Read the model definition and answer for the solid it produces. Units are mm, in the model's axes. A direction names the side the tool comes from. Coordinates: 2 decimals unless noted, no trailing zeros. Order: outer loops, then holes, each group sorted by start corner. A loop starts at its lowest first (then second) coordinate and runs counter-clockwise, first axis right, second up. Notation, with made-up numbers: (47.25, -7) -> (78.25, -7) arc R14 ccw to (78.25, 6) -> close; hole circle Ø8 at (39, -36.5). An arc over 180 degrees is marked (long way). Use CSV: the item, a comma, the result in double quotes.
```python
from build123d import *

# Parameters (mm, degrees)
F0_R     = 20
F0_R_2   = 1.5
F1_DEPTH = 7
F2_R     = 3.49999


# Not quite as in the source:
# - a fillet or chamfer is up to 0.001 mm smaller than in the source, because OpenCascade refuses the exact size


with BuildPart() as f1:
    # F0 (on Top) → F1 (new body)
    with BuildSketch(Plane.XY):
        Circle(F0_R)
        with BuildLine():
            Line((-11.2279220614, -9.9465454397), (-2.4047375097, -2.5430763869))
            ThreePointArc((-2.4047375097, -2.5430763869), (0, -3.5), (2.4047375097, -2.5430763869))
            Line((2.4047375097, -2.5430763869), (11.2279220614, -9.9465454397))
            ThreePointArc((11.2279220614, -9.9465454397), (0, -15), (-11.2279220614, -9.9465454397))
        make_face(mode=Mode.SUBTRACT)
        with BuildLine():
            ThreePointArc((-14.2279220614, -4.750393017), (-12.9903810568, 7.5), (-3, 14.6969384567))
            Line((-3, 14.6969384567), (-1, 3.3541019662))
            ThreePointArc((-1, 3.3541019662), (-3.0310889132, 1.75), (-3.4047375097, -0.8110255793))
            Line((-3.4047375097, -0.8110255793), (-14.2279220614, -4.750393017))
        make_face(mode=Mode.SUBTRACT)
        Circle(F0_R_2, mode=Mode.SUBTRACT)
        with BuildLine():
            ThreePointArc((3.4047375097, -0.8110255793), (3.0310889132, 1.75), (1, 3.3541019662))
            Line((1, 3.3541019662), (3, 14.6969384567))
            ThreePointArc((3, 14.6969384567), (12.9903810568, 7.5), (14.2279220614, -4.750393017))
            Line((14.2279220614, -4.750393017), (3.4047375097, -0.8110255793))
        make_face(mode=Mode.SUBTRACT)
    extrude(amount=F1_DEPTH)

    # F2 (radius 3.5 in the source; OpenCascade refuses exactly that, so slightly less here)
    f2_edges = [f1.edges().sort_by_distance(p)[0] for p in [
        (-20, 0, 7),
        (-20, 0, 0),
    ]]
    fillet(f2_edges, radius=F2_R)


solid = f1.part
```
Item 1: Find section A-A, the plane x = 0. Give the number of separate pieces and of enclosed holes in the cut face, then the cut area to 3 significant figures.
Return value:
separate pieces,"3"
enclosed holes,"0"
area,"168 mm^2"
Item 2: The mould has two halves that part along X. Classify faces 3 (the flat face through (-2.014, 9.105, 3.451)), 4 (the flat face through (0, 3, 0)): +X half, -X half, draft (parallel to the pull), parting line (faces both ways), or undercut.
Return value:
face 3,"undercut"
face 4,"draft"
Item 3: Find section C-C, the plane z = 6. Give the vertices of the cut face in (x, y), then the cut area to 3 significant figures.
Return value:
outline,"circle Ø37.9 at (0, 0); hole (-14.23, -4.75) -> (-3.4, -0.81) arc R3.5 cw to (-1, 3.35) -> (-3, 14.7) arc R15 ccw to start; hole (-11.23, -9.95) arc R15 ccw to (11.23, -9.95) -> (2.4, -2.54) arc R3.5 cw to (-2.4, -2.54) -> close; hole circle Ø3 at (0, 0); hole (1, 3.35) arc R3.5 cw to (3.4, -0.81) -> (14.23, -4.75) arc R15 ccw to (3, 14.7) -> close"
area,"592 mm^2"
Item 4: Straight lines are drawn through the part: line 1 along Y through (x, z) = (0, 3.25); line 2 along X through (y, z) = (9, 3.5); line 3 along Y through (x, z) = (-10, 3). For each, find the intervals that lie inside material, in ascending order.
Return value:
line 1,"y = -19.99 to -15, -3.5 to -1.5, 1.5 to 19.99"
line 2,"x = -17.86 to -12, -2 to 2, 12 to 17.86"
line 3,"y = -17.28 to -11.18, -8.92 to -3.21, 11.18 to 17.28"
Item 5: A tool of negligible diameter and unlimited length cuts with its end or side. For faces 1 (the flat face through (0, 3, 7)), 2 (the flat face through (-8.741, -2.753, 3.451)), from which of +Z, -Z, +X, -X, +Y, -Y can it reach the whole face along a straight path? Write none if from no direction.
Return value:
face 1,"+Z, +X, -X, +Y, -Y"
face 2,"+Z, -Z"
Item 6: Find section D-D, the plane z = 0.5. Give the vertices of the cut face in (x, y), then the cut area to 3 significant figures.
Return value:
outline,"circle Ø36.61 at (0, 0); hole (-14.23, -4.75) -> (-3.4, -0.81) arc R3.5 cw to (-1, 3.35) -> (-3, 14.7) arc R15 ccw to start; hole (-11.23, -9.95) arc R15 ccw to (11.23, -9.95) -> (2.4, -2.54) arc R3.5 cw to (-2.4, -2.54) -> close; hole circle Ø3 at (0, 0); hole (1, 3.35) arc R3.5 cw to (3.4, -0.81) -> (14.23, -4.75) arc R15 ccw to (3, 14.7) -> close"
area,"516 mm^2"
Item 7: Each of these flat-tipped pins is pushed along its axis until it touches: P1, Ø2, axis at x = -5, z = 5, coming from the +Y side; P2, Ø1.5, axis at x = 2.5, y = -5, coming from the -Z side; P3, Ø2, axis at x = 15.5, y = 9, coming from the -Z side; P4, Ø4, axis at x = -1, z = 2, coming from the +Y side. Where does it stop, or does it pass through?
Return value:
P1,"stops at y = 19.44"
P2,"passes through"
P3,"stops at z = 0.03"
P4,"stops at y = 20"
